from build123d import *

# Parameters (mm, degrees)
SKETCH1_R           = 1.25
SKETCH1_R_2         = 1.5
BOSS_EXTRUDE1_DEPTH = 5.72


with BuildPart() as part:
    # Sketch1 → Boss-Extrude1 (new body)
    with BuildSketch(Plane.XY):
        with BuildLine():
            Line((9.38, 23.147938931), (-1.036994756, 23.147938931))
            ThreePointArc((-1.036994756, 23.147938931), (-27.608078489, 10.53040656), (-0.142915981, 0))
            Line((-0.142915981, 0), (24.38, 0))
            Line((24.38, 0), (24.38, -10))
            Line((24.38, -10), (19.38, -10))
            Line((19.38, -10), (19.38, -15.72))
            Line((19.38, -15.72), (14.38, -15.72))
            Line((14.38, -15.72), (14.38, -9.950687023))
            Line((14.38, -9.950687023), (-1.62, -9.950687023))
            Line((-1.62, -9.950687023), (-1.62, -15.670687023))
            Line((-1.62, -15.670687023), (-6.62, -15.670687023))
            Line((-6.62, -15.670687023), (-6.62, -9.901374046))
            Line((-6.62, -9.901374046), (-22.62, -9.901374046))
            Line((-22.62, -9.901374046), (-22.62, -15.621374046))
            Line((-22.62, -15.621374046), (-27.62, -15.621374046))
            Line((-27.62, -15.621374046), (-27.62, -9.852061069))
            Line((-27.62, -9.852061069), (-32.62, -9.852061069))
            Line((-32.62, -9.852061069), (-32.62, 32.147938931))
            Line((-32.62, 32.147938931), (9.38, 32.147938931))
            Line((9.38, 32.147938931), (9.38, 23.147938931))
        make_face()
        with Locations((2.88, -7.950687023)):
            Circle(SKETCH1_R, mode=Mode.SUBTRACT)
        with Locations((-13.87, -7.901374046)):
            Circle(SKETCH1_R, mode=Mode.SUBTRACT)
        with Locations((3.879843111, -4.450687023)):
            Circle(SKETCH1_R_2, mode=Mode.SUBTRACT)
        with Locations((-27.12, -4.352061069)):
            Circle(SKETCH1_R_2, mode=Mode.SUBTRACT)
        with Locations((-27.12, 26.647938931)):
            Circle(SKETCH1_R_2, mode=Mode.SUBTRACT)
        with Locations((3.88, 26.647938931)):
            Circle(SKETCH1_R_2, mode=Mode.SUBTRACT)
    extrude(amount=BOSS_EXTRUDE1_DEPTH)


solid = part.part
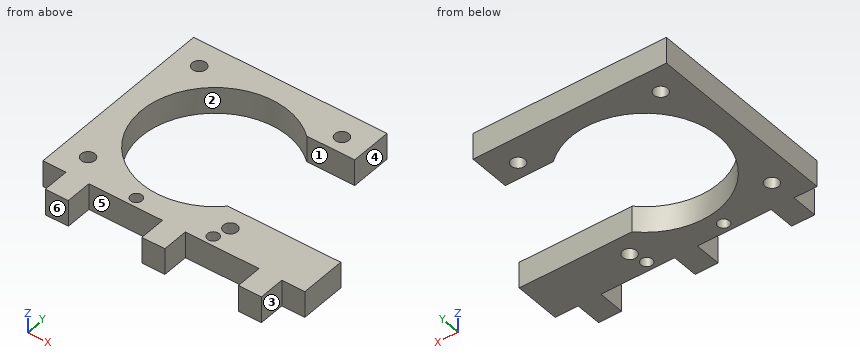
Build history of the part. All positions in model axes, mm. Face numbers are marked on the shaded views. A direction names the side the tool comes from. Coordinates: 2 decimals unless noted, no trailing zeros. Order: outer loops, then holes, each group sorted by start corner. A loop starts at its lowest first (then second) coordinate and runs counter-clockwise, first axis right, second up. Notation, with made-up numbers: (49.25, 13) -> (54.25, 13) arc R21 ccw to (54.25, 45) -> close; hole circle Ø7 at (20, 76.5). An arc over 180 degrees is marked (long way). One line per item, written item: value.
(1) Slice it at A-A, the plane x = -11.62. List the corners of the cut face in (y, z).
Checked values:
outline: (-9.9, 0) -> (-4.85, 0) -> (-4.85, 5.72) -> (-9.9, 5.72) -> close; (27.15, 0) -> (32.15, 0) -> (32.15, 5.72) -> (27.15, 5.72) -> close
(2) Drop flat-ended pins along their axis: pin 1 Ø1.7 at (x, z) = (2.5, 2) entering from -Y; pin 2 Ø2.5 at (x, z) = (-29, 3.5) entering from -Y. Give the stop position or say it passes through.
Checked values:
pin 1: y = -9.95
pin 2: y = -9.85
(3) Probe line 1 (X direction, y = -8, z = 2.7); line 2 (Y direction, x = -13.87, z = 4.35); line 3 (Y direction, x = 2.88, z = 4.4). List the from-to ranges inside material, lowest first. Write a range as [from, to].
Checked values:
line 1: [-32.62, -15.12], [-12.62, 1.63], [4.13, 24.38]
line 2: [-9.9, -9.15], [-6.65, -4.69], [26.99, 32.15]
line 3: [-9.95, -9.2], [-6.7, -5.57], [-3.33, 0], [23.15, 25.53], [27.77, 32.15]
(4) Mould opens along X. For the marked faces 1, 2 and 3 say: pulls with the +X half, pulls with the -X half, needs draft (parallel to the pull), parting line crosses it, or undercut.
Checked values:
face 1: needs draft
face 2: undercut
face 3: pulls with the +X half
(5) Tool access for the marked faces 4, 5 and 6: list every direction of +Z, -Z, +X, -X, +Y, -Y with a clear straight run to the whole face (end or side of a thin tool).
Checked values:
face 4: +Z, -Z, +X, +Y
face 5: +Z, -Z, -Y
face 6: +Z, -Z, -X, -Y
(6) Slice it at B-B, the plane x = 8.5. List the corners of the cut face in (y, z).
Checked values:
outline: (-9.95, 0) -> (0, 0) -> (0, 5.72) -> (-9.95, 5.72) -> close; (23.15, 0) -> (32.15, 0) -> (32.15, 5.72) -> (23.15, 5.72) -> close
(7) Slice it at D-D, the plane x = 18. List the corners of the cut face in (y, z), plus the area to 3 significant figures.
Checked values:
outline: (-15.72, 0) -> (0, 0) -> (0, 5.72) -> (-15.72, 5.72) -> close
area: 89.9 mm2
(8) Slice it at C-C, the plane z = 5.05. List the corners of the cut face in (x, y).
Checked values:
outline: (-32.62, -9.85) -> (-27.62, -9.85) -> (-27.62, -15.62) -> (-22.62, -15.62) -> (-22.62, -9.9) -> (-6.62, -9.9) -> (-6.62, -15.67) -> (-1.62, -15.67) -> (-1.62, -9.95) -> (14.38, -9.95) -> (14.38, -15.72) -> (19.38, -15.72) -> (19.38, -10) -> (24.38, -10) -> (24.38, 0) -> (-0.14, 0) arc R16 cw (long way) to (-1.04, 23.15) -> (9.38, 23.15) -> (9.38, 32.15) -> (-32.62, 32.15) -> close; hole circle Ø3 at (-27.12, -4.35); hole circle Ø3 at (-27.12, 26.65); hole circle Ø2.5 at (-13.87, -7.9); hole circle Ø2.5 at (2.88, -7.95); hole circle Ø3 at (3.88, -4.45); hole circle Ø3 at (3.88, 26.65)
